Verification items for the finished model (mm, model axes). A direction names the side the tool comes from. Coordinates: 2 decimals unless noted, no trailing zeros. Order: outer loops, then holes, each group sorted by start corner. A loop starts at its lowest first (then second) coordinate and runs counter-clockwise, first axis right, second up. Notation, with made-up numbers: M 50.25,-39.5 L 66.25,-39.5 A17 cw 66.25,-28.5 Z; hole C -15.5,71.25 d10. An arc over 180 degrees is marked long. Use one line per item in the form item = value. Start each with the question number.
```python
from build123d import *

# Parameters (mm, degrees)
SKETCH1_W           = 35
SKETCH1_H           = 20.6
BOSS_EXTRUDE1_DEPTH = 1.5
SKETCH1_3_R         = 1.75
BOSS_EXTRUDE2_DEPTH = 8
CUT_EXTRUDE1_START  = 3
SKETCH1_5_R         = 3.75
CUT_EXTRUDE1_DEPTH  = 27.094673052
FILLET1_R           = 5


with BuildPart() as part:
    # Sketch1 → Boss-Extrude1 (new body)
    with BuildSketch(Plane(origin=(0, 0, 0), x_dir=(1, 0, 0), z_dir=(0, 1, 0))):
        Rectangle(SKETCH1_W, SKETCH1_H)
        with BuildLine():
            Line((-17.5, -10.3), (-17.040552602, -10.3))
            ThreePointArc((-17.040552602, -10.3), (-17.010151892, -10.025746493), (-17, -9.75))
            ThreePointArc((-17, -9.75), (-17.127155813, -8.781754163), (-17.5, -7.879171307))
            Line((-17.5, -7.879171307), (-17.5, -10.3))
        make_face()
        with BuildLine():
            ThreePointArc((17.040552602, 10.3), (17.065766034, 9.050771792), (17.5, 7.879171307))
            Line((17.5, 7.879171307), (17.5, 10.3))
            Line((17.5, 10.3), (17.040552602, 10.3))
        make_face()
    extrude(amount=BOSS_EXTRUDE1_DEPTH)

    # Sketch1<3> → Boss-Extrude2 (add)
    with BuildSketch(Plane(origin=(0, 0, 0), x_dir=(1, 0, 0), z_dir=(0, 1, 0))):
        with BuildLine():
            Line((-17.5, -10.3), (-17.5, -2))
            Line((-17.5, -2), (-19, -2))
            Line((-19, -2), (-19, -6.43337521))
            ThreePointArc((-19, -6.43337521), (-24.380199188, -10.690294559), (-17.609936306, -11.8))
            Line((-17.609936306, -11.8), (19, -11.8))
            Line((19, -11.8), (19, 6.43337521))
            ThreePointArc((19, 6.43337521), (24.380199188, 10.690294559), (17.609936306, 11.8))
            Line((17.609936306, 11.8), (-19, 11.8))
            Line((-19, 11.8), (-19, 10.3))
            Line((-19, 10.3), (17.5, 10.3))
            Line((17.5, 10.3), (17.5, -10.3))
            Line((17.5, -10.3), (-17.5, -10.3))
        make_face()
        with Locations(Location((-20.75, -9.75, 0), (0, 0, 270))):
            Circle(SKETCH1_3_R, mode=Mode.SUBTRACT)
        with Locations(Location((20.75, 9.75, 0), (0, 0, 270))):
            Circle(SKETCH1_3_R, mode=Mode.SUBTRACT)
    extrude(amount=BOSS_EXTRUDE2_DEPTH)

    # Sketch1<5> → Cut-Extrude1 (cut, through all)
    with BuildSketch(Plane(origin=(0, 0, 0), x_dir=(1, 0, 0), z_dir=(0, 1, 0)).offset(CUT_EXTRUDE1_START)):
        with Locations((20.75, 9.75)):
            Circle(SKETCH1_5_R)
        with Locations((-20.75, -9.75)):
            Circle(SKETCH1_5_R)
    extrude(amount=CUT_EXTRUDE1_DEPTH, mode=Mode.SUBTRACT)

    # Fillet1
    # the kernel refuses this fillet: 5 mm, written as the material it adds along each edge
    with BuildSketch(Plane(origin=(-19, 0, 6.43337521), x_dir=(-0.9985759338365271, 0, -0.05334889279551997), z_dir=(0, 1, 0))) as fillet1_piece_1:
        with BuildLine():
            CenterArc((5.235232079, -4.540349679), FILLET1_R, 114.760021094, 63.94168422)
            Line((0.236515659, -4.42706179), (0, 0))
            ThreePointArc((0, 0), (1.570569624, -0.34473774), (3.141139248, 0))
        make_face()
    extrude(amount=3)
    with BuildSketch(Plane(origin=(-17.609936306, 0, 11.8), x_dir=(-0.6872011618867198, 0, 0.7264671796451251), z_dir=(0, 1, 0))) as fillet1_piece_2:
        with BuildLine():
            CenterArc((2.228659001, 4.919887463), FILLET1_R, 223.40896289, 36.320705761)
            Line((-1.403676897, 1.483881654), (0, 0))
            ThreePointArc((0, 0), (0.6685977, 0.060084403), (1.337195401, 0))
        make_face()
    extrude(amount=3)
    with BuildSketch(Plane(origin=(17.609936306, 0, -11.8), x_dir=(-1, 0, 0), z_dir=(0, 1, 0))) as fillet1_piece_3:
        with BuildLine():
            CenterArc((2.042599714, -5), FILLET1_R, 90, 36.320705761)
            ThreePointArc((-0.918922233, -0.971428571), (-0.41581177, -0.527004357), (0, 0))
            Line((0, 0), (2.042599714, 0))
        make_face()
    extrude(amount=3)
    with BuildSketch(Plane(origin=(19, 0, -6.43337521), x_dir=(0.9986229541246332, 0, 0.052461371459300826), z_dir=(0, 1, 0))) as fillet1_piece_4:
        with BuildLine():
            CenterArc((5.245318282, -4.538486728), FILLET1_R, 114.810943637, 68.196252011)
            Line((0.252203511, -4.800793585), (0, 0))
            ThreePointArc((0, 0), (1.573595485, -0.346134954), (3.147190969, 0))
        make_face()
    extrude(amount=3)


solid = part.part
```
1. Cross-section at C-C on y = 2. Enter the section's corners in (x, z), and give its area (3 significant figures).
2. Release check for a two-part mould opening along X. For faces 6 (the flat face through (17.5, 5, 0)), 7 (the cylindrical face through (-17.1, 1.48, 12.04)), 8 (the flat face through (-19, 5, 4)) record: pulls with the +X half, pulls with the -X half, needs draft (parallel to the pull), parting line crosses it, or undercut.
3. Cross-section at D-D on x = 20.75. Enter the section's corners in (y, z), and give its area (3 significant figures).
4. Cross-section at B-B on y = 7. Enter the section's corners in (x, z).
5. Material ranges on line 1 along X through (y, z) = (2.05, 9.75); line 2 along X through (y, z) = (1.8, -9.75); line 3 along X through (y, z) = (1.15, 9.75), recorded low to high.
6. Depth check by flat-ended pin: P1, Ø1.2, axis at x = -18.5, y = 5, coming from the -Z side; P2, Ø3, axis at x = 20.75, z = -9.75, coming from the +Y side; P3, Ø1, axis at x = 6, y = 2.5, coming from the +Z side; P4, Ø2.5, axis at y = 5.5, z = 3.5, coming from the +X side. Enter the tip coordinate at first touch or a pass-through.
7. Tool access check on faces 1 (the cylindrical face through (17.248, 5.465, -11.091)), 2 (the flat face through (-17.5, 1, -4)), 3 (the flat face through (-17.5, 5, 5)), 4 (the flat face through (-19, 4, -11)), 5 (the cylindrical face through (-24.07, 1.48, 11.49)). Record the directions out of +Z, -Z, +X, -X, +Y, -Y that give a thin tool (end or side, any length) a straight path to the whole face; none if there is none.
8. Cross-section at A-A on z = -9.75. Enter the section's corners in (x, y).
Final values:
q1.outline = M -22.14,6.27 A5 cw -19,2 L -17.5,2 L -17.5,10.3 L 17.5,10.3 L 17.5,-10.3 L -19,-10.3 L -19,-11.8 L 15.57,-11.8 A5 cw 18.53,-12.77 A3.75 ccw long 22.14,-6.27 A5 cw 19,-1.63 L 19,11.8 L -15.57,11.8 A5 cw -18.53,12.77 A3.75 ccw long Z; hole C -20.75,9.75 d3.5; hole C 20.75,-9.75 d3.5
q1.area = 218 mm2
q2.face_6 = undercut
q2.face_7 = pulls with the +X half
q2.face_8 = pulls with the -X half
q3.outline = M 0,-13.5 L 3,-13.5 L 3,-11.5 L 0,-11.5 Z; M 0,-8 L 3,-8 L 3,-5.43 L 0,-5.43 Z
q3.area = 13.7 mm2
q4.outline = M -19,-11.8 L 17.61,-11.8 A3.75 cw 17.04,-10.3 L -19,-10.3 Z; M -19,2 L -17.5,2 L -17.5,7.88 A3.75 cw -19,6.43 Z; M -17.61,11.8 A3.75 cw -17.04,10.3 L 17.5,10.3 L 17.5,-7.88 A3.75 cw 19,-6.43 L 19,11.8 Z
q5.line_1 = -24.5 to -22.5, -19 to -17.5, 17.5 to 19
q5.line_2 = 17.5 to 19, 22.5 to 24.5
q5.line_3 = -24.5 to -22.5, -19 to 19
q6.P1 = -11.8
q6.P2 = through
q6.P3 = 11.8
q6.P4 = 19
q7.face_1 = +X, +Y
q7.face_2 = -X, +Y, -Y
q7.face_3 = +Y
q7.face_4 = -Z, -X, +Y, -Y
q7.face_5 = +Y, -Y
q8.outline = M -17.5,0 L 19,0 L 19,3 L 17.5,3 L 17.5,1.5 L -17.5,1.5 Z; M 22.5,0 L 24.5,0 L 24.5,3 L 22.5,3 Z
